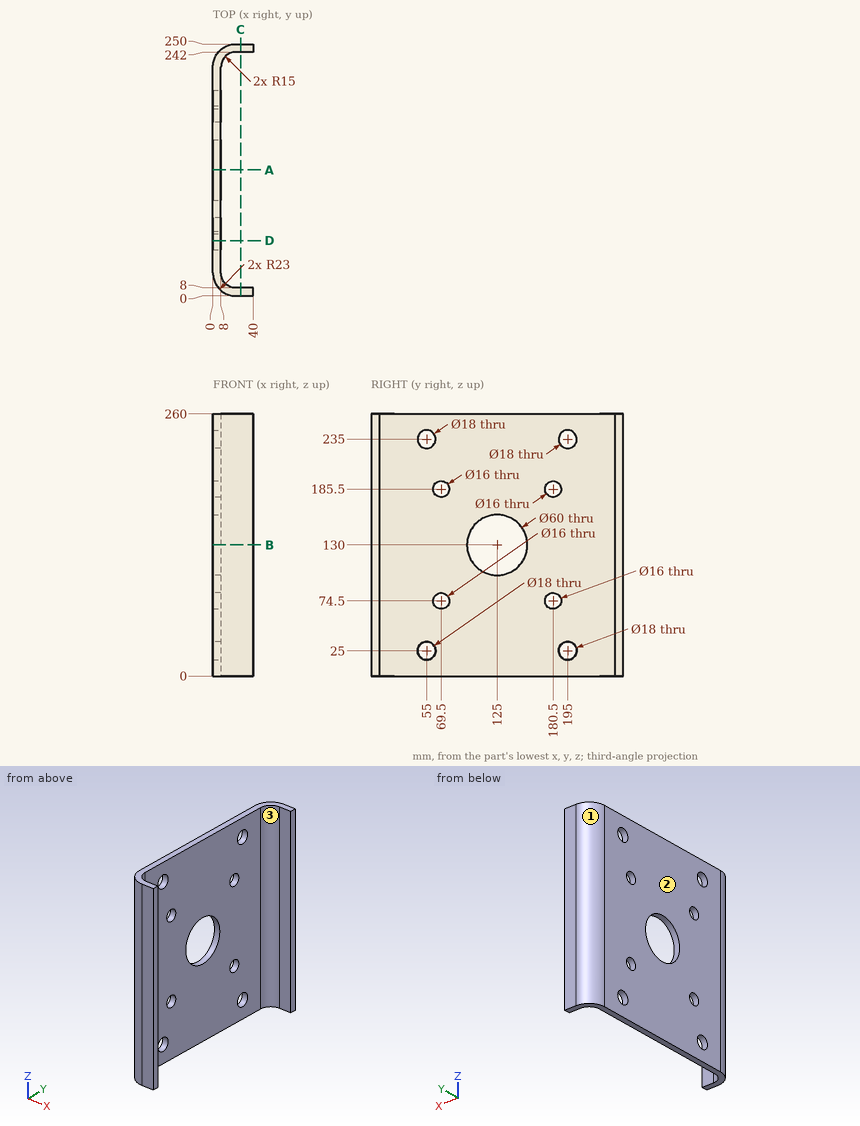
Geometry check sheet. Reference: drawing and pictorial views, mm from the part's lowest x, y, z. Round coordinates to 2 decimals unless told otherwise and drop trailing zeros. Write each loop counter-clockwise with the first axis right and the second up, starting at its lowest first coordinate (ties: lowest second). Pieces come first, ordered by that corner, then holes.
Item 1: Section check A-A (y = 125). Record the boundary of the cut face in (x, z), plus the area to 3 significant figures.
Determined:
outline: (0, 0) - (8, 0) - (8, 100) - (0, 100) - close; (0, 160) - (8, 160) - (8, 260) - (0, 260) - close
area: 1,600 mm2
Item 2: Material ranges on line 1 along Z through (x, y) = (7, 181); line 2 along Y through (x, z) = (3.75, 25); line 3 along Y through (x, z) = (4, 25), recorded low to high.
Determined:
line 1: z = 0 to 66.52, 82.48 to 177.52, 193.48 to 260
line 2: y = 10.41 to 46, 64 to 186, 204 to 239.59
line 3: y = 10.04 to 46, 64 to 186, 204 to 239.96
Item 3: Section check D-D (y = 55). Record the boundary of the cut face in (x, z).
Determined:
outline: (0, 0) - (8, 0) - (8, 16) - (0, 16) - close; (0, 34) - (8, 34) - (8, 226) - (0, 226) - close; (0, 244) - (8, 244) - (8, 260) - (0, 260) - close
Item 4: Section check C-C (x = 27.5). Record the boundary of the cut face in (y, z).
Determined:
outline: (0, 0) - (8, 0) - (8, 260) - (0, 260) - close; (242, 0) - (250, 0) - (250, 260) - (242, 260) - close
Item 5: Mould release check, pull along Y, two halves, no side actions. Record for the marked faces 1, 2 and 3: +Y half, -Y half, draft (parallel to the pull), parting line (faces both ways), or undercut.
Determined:
face 1: +Y half
face 2: draft
face 3: undercut
Item 6: Section check B-B (z = 130). Record the boundary of the cut face in (x, y).
Determined:
outline: (0, 23) arc R23 ccw to (23, 0) - (40, 0) - (40, 8) - (23, 8) arc R15 cw to (8, 23) - (8, 95) - (0, 95) - close; (0, 155) - (8, 155) - (8, 227) arc R15 cw to (23, 242) - (40, 242) - (40, 250) - (23, 250) arc R23 ccw to (0, 227) - close
Item 7: Go/stop test with flat-tipped pins: pin 1 Ø10 at (y, z) = (55, 34) entering from +X; pin 2 Ø18.5 at (y, z) = (180.5, 74.5) entering from -X; pin 3 Ø12 at (x, z) = (16, 98) entering from +Y; pin 4 Ø3 at (x, z) = (7.5, 102) entering from -Y. Record where each tip stops, or that it passes through.
Determined:
pin 1: stops at x = 8
pin 2: stops at x = 0
pin 3: stops at y = 249.98
pin 4: stops at y = 4.75
